Input: part model. Units: mm. Frame: model coordinates. Round coordinates to 2 decimals unless told otherwise and drop trailing zeros. Loops run counter-clockwise (first coordinate to the right, second up) from the corner with the lowest first, then second, coordinate; pieces in that order, holes last. Notation, with made-up numbers: M 40.5,24.5 L 73.5,24.5 A25 cw 73.5,40.5 Z; hole C -19,-24 d4. An arc over 180 degrees is marked long. Put each result on its own line as item: value. Start each with the question number.
1) Section B-B on z = -13.97. Output: boundary loops of the cut face in (x, y) (3 decimals).
2) Pin query (flat end, axial travel): pin 1 (0.7 mm diameter, centred on y = 2, z = -4.5, fed in from -X) (3 decimals); pin 2 (2.5 mm diameter, centred on x = 31.75, z = -9.525, fed in from +Y); pin 3 (1.5 mm diameter, centred on x = 26.5, y = 2, fed in from +Z). Return the tip coordinate at first contact, or that it passes through.
3) Line query: probe 1 along Y at (x, z) = (7.5, -5.08) (3 decimals); probe 2 along X at (y, z) = (1.4, -9.5); probe 3 along X at (y, z) = (0.65, -4.5) (3 decimals). Output: solid intervals per line, ascending.
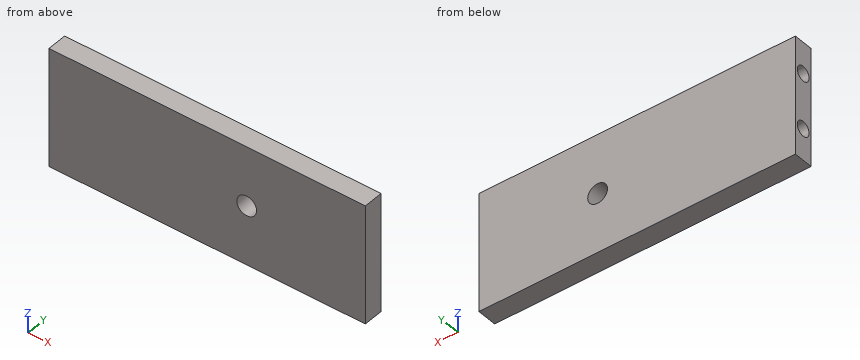
from build123d import *

# Parameters (mm, degrees)
SKETCH1_W           = 50.8
SKETCH1_H           = 19.05
BOSS_EXTRUDE1_DEPTH = 3.175
SKETCH2_R           = 1.190625
CUT_EXTRUDE1_DEPTH  = 9.525
SKETCH3_R           = 1.5875
CUT_EXTRUDE2_DEPTH  = 55.34724579


with BuildPart() as part:
    # Sketch1 → Boss-Extrude1 (new body)
    with BuildSketch(Plane(origin=(0, 0, 0), x_dir=(1, 0, 0), z_dir=(0, 1, 0))):
        with Locations((25.4, 9.525)):
            Rectangle(SKETCH1_W, SKETCH1_H)
    extrude(amount=BOSS_EXTRUDE1_DEPTH)

    # Sketch2 → Cut-Extrude1 (cut)
    with BuildSketch(Plane.ZY):
        with Locations((-5.08, 1.5875)):
            Circle(SKETCH2_R)
        with Locations((-13.97, 1.5875)):
            Circle(SKETCH2_R)
    extrude(amount=-CUT_EXTRUDE1_DEPTH, mode=Mode.SUBTRACT)

    # Sketch3 → Cut-Extrude2 (cut, through all)
    with BuildSketch(Plane(origin=(0, 3.175, 0), x_dir=(1, 0, 0), z_dir=(0, 1, 0))):
        with Locations(Location((31.75, 9.525, 0), (0, 0, 270))):
            Circle(SKETCH3_R)
    extrude(amount=-CUT_EXTRUDE2_DEPTH, mode=Mode.SUBTRACT)


solid = part.part
Geometry results:
1. outline: M 0,0 L 50.8,0 L 50.8,3.175 L 0,3.175 L 0,2.778 L 9.525,2.778 L 9.525,0.397 L 0,0.397 Z
2. pin 1: stops at x = 9.525
2. pin 2: passes through
2. pin 3: stops at z = 0
3. probe 1: y = 0 to 0.397, 2.778 to 3.175
3. probe 2: x = 0 to 30.16, 33.34 to 50.8
3. probe 3: x = 9.525 to 50.8
